```python
from build123d import *

# Parameters (mm, degrees)
F0_R     = 13
F1_DEPTH = 40
F2_R     = 4
F3_DEPTH = 13
F4_SIZE  = 1
F6_DEPTH = 4
F8_DEPTH = 25


with BuildPart() as f1:
    # F0 (on Right) → F1 (new body, symmetric)
    with BuildSketch(Plane.YZ):
        Circle(F0_R)
    extrude(amount=F1_DEPTH, both=True)

    # F2 (on Top) → F3 (cut, symmetric)
    with BuildSketch(Plane.XY):
        Circle(F2_R)
    extrude(amount=F3_DEPTH, both=True, mode=Mode.SUBTRACT)

    # F4
    f4_edges = [f1.edges().sort_by_distance(p)[0] for p in [
        (-40, -13, 0),
        (40, -13, 0),
    ]]
    chamfer(f4_edges, length=F4_SIZE)

    # F5 (on Front) → F6 (cut, symmetric)
    with BuildSketch(Plane.XZ):
        with BuildLine():
            Line((39, 13), (0, 13))
            ThreePointArc((0, 13), (7.0943058496, 9.2829175487), (15, 8))
            Line((15, 8), (40, 8))
            Line((40, 8), (40, 12))
            Line((40, 12), (39, 13))
        make_face()
    extrude(amount=F6_DEPTH, both=True, mode=Mode.SUBTRACT)

    # F7 (on face) → F8 (cut)
    with BuildSketch(Plane.YZ.offset(40)):
        with BuildLine():
            ThreePointArc((5.3934227849, 11.8283976372), (4.7044921415, 12.1189006799), (4, 12.3693168769))
            Line((4, 12.3693168769), (4, 8))
            Line((4, 8), (5.3934227849, 11.8283976372))
        make_face()
        with BuildLine():
            Line((-5.3934227849, 11.8283976372), (-4, 8))
            Line((-4, 8), (-4, 12.3693168769))
            ThreePointArc((-4, 12.3693168769), (-4.7044921415, 12.1189006799), (-5.3934227849, 11.8283976372))
        make_face()
    extrude(amount=-F8_DEPTH, mode=Mode.SUBTRACT)


solid = f1.part
```
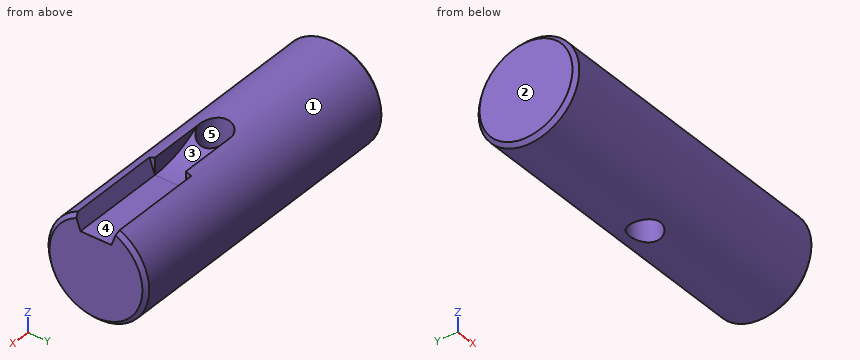
The model under review builds one solid part; all positions refer to its coordinate system, in mm. Face numbers are marked on the shaded views. A direction names the side the tool comes from. Round coordinates to 2 decimals unless told otherwise and drop trailing zeros. Loops run counter-clockwise (first coordinate to the right, second up) from the corner with the lowest first, then second, coordinate; pieces in that order, holes last. Notation, with made-up numbers: (-29, 70.25) - (9, 70.25) arc R5 cw to (9, 77.25) - close; hole circle Ø11 at (-27.75, -13). An arc over 180 degrees is marked (long way). Write each question's results on one line, items separated by ' | '. Start each with the question number.
Q1. Tool access review of the marked faces 4 and 5: name each direction out of +Z, -Z, +X, -X, +Y, -Y from which nothing blocks a thin tool from reaching the whole face with its end or side.
Q2. Insertion check: P1, Ø1, axis at x = -17, z = 5.5, coming from the +Y side; P2, Ø5, axis at x = 4.5, z = 11, coming from the +Y side; P3, Ø1.5, axis at x = -30.5, z = -8.5, coming from the +Y side. Each pin has a flat end and moves straight along its axis. Give the tip position at first contact, or say it passes through.
Q3. Take a section at B-B on y = 0. Give the boundary of the cut face in (x, z), plus the area to 3 significant figures.
Q4. Draft analysis for pull direction Y (two halves, no side actions). For the marked faces 1, 2 and 3, state which applies: pulls with the +Y half, pulls with the -Y half, needs draft (parallel to the pull), parting line crosses it, or undercut.
Q5. Take a section at D-D on x = 0. Give the boundary of the cut face in (y, z).
Q6. Take a section at C-C on x = -19.5. Give the boundary of the cut face in (y, z).
Q7. Wall thickness on line 1 along Y through (x, z) = (0, -0.5); line 2 along X through (y, z) = (0, -1.75); line 3 along X through (y, z) = (1.5, 5.75): over which ranges is each line inside the solid? List them lowest first. Write a range as [from, to].
Q8. Take a section at A-A on z = 0. Give the boundary of the cut face in (x, y), plus the area to 3 significant figures.
Data:
1) face 4: +Z, +X | face 5: +Z, -Z
2) P1: stops at y = 12 | P2: stops at y = 9.84 | P3: stops at y = 10.44
3) outline: (-40, -12) - (-39, -13) - (-4, -13) - (-4, 13) - (-39, 13) - (-40, 12) - close; (4, -13) - (39, -13) - (40, -12) - (40, 8) - (15, 8) arc R25 cw to (4, 10.55) - close | area: 1,700 mm²
4) face 1: parting line crosses it | face 2: needs draft | face 3: undercut
5) outline: (-4, -12.37) - (-4, 12.37) arc R13 ccw to start; (4, -12.37) arc R13 ccw to (4, 12.37) - close
6) outline: circle Ø26 at (0, 0)
7) line 1: y = [-12.99, -4], [4, 12.99] | line 2: x = [-40, -4], [4, 40] | line 3: x = [-40, -3.71], [3.71, 40]
8) outline: (-40, -12) - (-39, -13) - (39, -13) - (40, -12) - (40, 12) - (39, 13) - (-39, 13) - (-40, 12) - close; hole circle Ø8 at (0, 0) | area: 2,030 mm²
